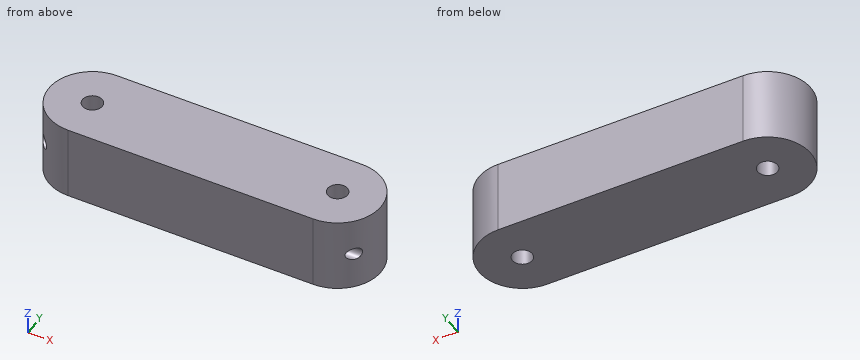
from build123d import *

# Parameters (mm, degrees)
BOSS_EXTRUDE1_DEPTH = 6
SKETCH2_R           = 1.6
CUT_EXTRUDE1_DEPTH  = 50.010203019
SKETCH3_R           = 1
CUT_EXTRUDE2_DEPTH  = 60


with BuildPart() as part:
    # Sketch1 → Boss-Extrude1 (new, symmetric)
    with BuildSketch(Plane.XY):
        with BuildLine():
            Line((0, 7), (40, 7))
            ThreePointArc((40, 7), (47, 0), (40, -7))
            Line((40, -7), (0, -7))
            ThreePointArc((0, -7), (-7, 0), (0, 7))
        make_face()
    extrude(amount=BOSS_EXTRUDE1_DEPTH, both=True)

    # Sketch2 → Cut-Extrude1 (cut, through all)
    with BuildSketch(Plane.XY.offset(6)):
        Circle(SKETCH2_R)
        with Locations((40, 0)):
            Circle(SKETCH2_R)
    extrude(amount=-CUT_EXTRUDE1_DEPTH, mode=Mode.SUBTRACT)

    # Sketch3 → Cut-Extrude2 (cut, symmetric)
    with BuildSketch(Plane(origin=(0, 0, 0), x_dir=(0, 0, -1), z_dir=(1, 0, 0))):
        with Locations((0, -4.5)):
            Circle(SKETCH3_R)
    extrude(amount=CUT_EXTRUDE2_DEPTH, both=True, mode=Mode.SUBTRACT)


solid = part.part
Source: CAD feature listing. Evaluate the final solid. Frame: model axes, mm. Round coordinates to 2 decimals unless told otherwise and drop trailing zeros. Loops run counter-clockwise (first coordinate to the right, second up) from the corner with the lowest first, then second, coordinate; pieces in that order, holes last. Notation, with made-up numbers: (12, 86.5) - (21, 86.5) arc R20 ccw to (21, 91.5) - close; hole circle Ø3 at (34.25, 69). An arc over 180 degrees is marked (long way). Write item = value, one per line. Start each with the question number.
(1) Ray query, line 1 along Y through (x, z) = (34.5, 0); line 2 along Y through (x, z) = (0, 3.5); line 3 along X through (y, z) = (-0.75, 3.75). Return the intervals inside material, ascending. Write a range as from..to.
(2) Section query D-D, the plane z = 4. Output: boundary loops of the cut face in (x, y).
(3) Section query C-C, the plane z = 0. Output: boundary loops of the cut face in (x, y), plus the area to 3 significant figures.
(4) Section query B-B, the plane x = 40.5. Output: boundary loops of the cut face in (y, z), plus the area to 3 significant figures.
(5) Pin query (flat end, axial travel): pin 1 (5 mm diameter, centred on y = -5, z = -2, fed in from +X). Return the tip coordinate at first contact, or that it passes through.
(6) Section query A-A, the plane y = 0. Output: boundary loops of the cut face in (x, z), plus the area to 3 significant figures.
Conclusion:
q1.line_1 = -7..-5.5, -3.5..7
q1.line_2 = -7..-1.6, 1.6..7
q1.line_3 = -6.96..-1.41, 1.41..38.59, 41.41..46.96
q2.outline = (0, -7) - (40, -7) arc R7 ccw to (40, 7) - (0, 7) arc R7 ccw to start; hole circle Ø3.2 at (0, 0); hole circle Ø3.2 at (40, 0)
q3.outline = (-6.06, -3.5) - (46.06, -3.5) arc R7 ccw to (40, 7) - (0, 7) arc R7 ccw to start; (-4.33, -5.5) arc R7 ccw to (0, -7) - (40, -7) arc R7 ccw to (44.33, -5.5) - close; hole circle Ø3.2 at (0, 0); hole circle Ø3.2 at (40, 0)
q3.area = 597 mm2
q4.outline = (-6.98, -6) - (-1.52, -6) - (-1.52, 6) - (-6.98, 6) - close; (1.52, -6) - (6.98, -6) - (6.98, 6) - (1.52, 6) - close; hole circle Ø2 at (-4.5, 0)
q4.area = 128 mm2
q5.pin_1 = 46.54
q6.outline = (-7, -6) - (-1.6, -6) - (-1.6, 6) - (-7, 6) - close; (1.6, -6) - (38.4, -6) - (38.4, 6) - (1.6, 6) - close; (41.6, -6) - (47, -6) - (47, 6) - (41.6, 6) - close
q6.area = 571 mm2
